The listing builds one solid part. Answer for the finished solid, in the listing's coordinates (mm). A direction names the side the tool comes from. Round coordinates to 2 decimals unless told otherwise and drop trailing zeros. Write each loop counter-clockwise with the first axis right and the second up, starting at its lowest first coordinate (ties: lowest second). Pieces come first, ordered by that corner, then holes.
Item 1: Each of these flat-tipped pins is pushed along its axis until it touches: pin 1 (1.5 mm diameter, centred on x = -9, z = 5, fed in from -Y); pin 2 (2 mm diameter, centred on y = 1.5, z = 5, fed in from -X); pin 3 (3.5 mm diameter, centred on x = 0, z = 0, fed in from -Y); pin 4 (1 mm diameter, centred on x = 5.5, y = 1, fed in from -Z). Where does it stop, or does it pass through?
Item 2: Find section A-A on x = 0. Give the vertices of the cut face in (y, z).
Item 3: Find section B-B on z = 0. Give the vertices of the cut face in (x, y), then the cut area to 3 significant figures.
Item 4: For a pull along X with two mould halves and no side action, classify faces 3 (the face through (3, 4, 0)), 4 (the face through (12.932, 2.226, 5.362)), 5 (the face through (-2.15, 2.03, -0.09)) as +X half, -X half, draft (parallel to the pull), parting line (faces both ways), or undercut.
Item 5: Find section D-D on z = 3.5. Give the vertices of the cut face in (x, y), then the cut area to 3 significant figures.
Item 6: Find the intervals of material crossed by probe 1 along Z at (x, y) = (0, 2.6); probe 2 along Y at (x, z) = (7.25, 9), in increasing order.
Item 7: A tool of negligible diameter and unlimited length cuts with its end or side. For faces 1 (the face through (-2, 0, -2)), 2 (the face through (-5.158, 0.246, -3.955)), from which of +Z, -Z, +X, -X, +Y, -Y can it reach the whole face along a straight path? Write none if from no direction.
Item 8: Find section C-C on y = 3.6. Give the vertices of the cut face in (x, z), then the cut area to 3 significant figures.
```python
from build123d import *

# Parameters (mm, degrees)
SKETCH1_R           = 14
BOSS_EXTRUDE1_DEPTH = 4
SKETCH2_R           = 14
SKETCH2_R_2         = 6.5
CUT_EXTRUDE1_DEPTH  = 0.5
SKETCH3_R           = 2.15
CUT_EXTRUDE2_DEPTH  = 4


with BuildPart() as part:
    # Sketch1 → Boss-Extrude1 (new body)
    with BuildSketch(Plane(origin=(0, 0, 0), x_dir=(1, 0, 0), z_dir=(0, 1, 0))):
        Circle(SKETCH1_R)
    extrude(amount=BOSS_EXTRUDE1_DEPTH)

    # Sketch2 → Cut-Extrude1 (cut)
    with BuildSketch(Plane.XZ):
        Circle(SKETCH2_R)
        Circle(SKETCH2_R_2, mode=Mode.SUBTRACT)
    extrude(amount=-CUT_EXTRUDE1_DEPTH, mode=Mode.SUBTRACT)

    # Sketch3 → Cut-Extrude2 (cut)
    with BuildSketch(Plane(origin=(0, 4, 0), x_dir=(1, 0, 0), z_dir=(0, 1, 0))):
        Circle(SKETCH3_R)
    extrude(amount=-CUT_EXTRUDE2_DEPTH, mode=Mode.SUBTRACT)


solid = part.part
```
Check values:
1. pin 1: stops at y = 0.5
1. pin 2: stops at x = -13.42
1. pin 3: passes through
1. pin 4: stops at z = -13.08
2. outline: (0, -6.5) - (0.5, -6.5) - (0.5, -14) - (4, -14) - (4, -2.15) - (0, -2.15) - close; (0, 2.15) - (4, 2.15) - (4, 14) - (0.5, 14) - (0.5, 6.5) - (0, 6.5) - close
3. outline: (-14, 0.5) - (-6.5, 0.5) - (-6.5, 0) - (-2.15, 0) - (-2.15, 4) - (-14, 4) - close; (2.15, 0) - (6.5, 0) - (6.5, 0.5) - (14, 0.5) - (14, 4) - (2.15, 4) - close
3. area: 87.3 mm2
4. face 3: draft
4. face 4: parting line
4. face 5: undercut
5. outline: (-13.56, 0.5) - (-5.48, 0.5) - (-5.48, 0) - (5.48, 0) - (5.48, 0.5) - (13.56, 0.5) - (13.56, 4) - (-13.56, 4) - close
5. area: 100 mm2
6. probe 1: z = -14 to -2.15, 2.15 to 14
6. probe 2: y = 0.5 to 4
7. face 1: +Z, -Z, +X, -X, -Y
7. face 2: -Y
8. outline: circle Ø28 at (0, 0); hole circle Ø4.3 at (0, 0)
8. area: 601 mm2
